Autodesk Inventor part; units mm, degrees
ref_plane "YZ Plane" through (0, 0, 0) normal (1, 0, 0) x (0, 1, 0)
ref_plane "XZ Plane" through (0, 0, 0) normal (0, 1, 0) x (-1, 0, 0)
ref_plane "XY Plane" through (0, 0, 0) normal (0, 0, 1) x (1, 0, 0)
sketch "Boceto1" plane through (0, 0, 0) normal (0, 0, 1) x (1, 0, 0)
  line L0 (0, 0) -> (0, 30.8)
  line L1 (0, 30.8) -> (7, 30.8)
  line L2 (7, 30.8) -> (7, 20.8)
  line L3 (0, 0) -> (45, 0)
  line L4 (45, 0) -> (45, 4.6)
  line L5 (45, 4.6) -> (17, 4.6)
  line L6 (17, 4.6) -> (7, 20.8)
  dimension "d0" = 30.8
  dimension "d1" = 7
  dimension "d2" = 10
  dimension "d3" = 45
  dimension "d4" = 4.6
  dimension "d5" = 28
extrude "Extrusión1" add sketch "Boceto1" along normal blind 1.8
sketch "Boceto2" plane through (0, 0, 1.8) normal (0, 0, 1) x (1, 0, 0)
  line L0 (0, 0) -> (0, 30.8)
  line L1 (45, 0) -> (0, 0)
  line L2 (45, 4.6) -> (45, 0)
  line L3 (17, 4.6) -> (45, 4.6)
  line L4 (7, 30.8) -> (7, 20.8)
  line L5 (17, 4.6) -> (7, 4.6)
  line L6 (0, 6.8) -> (7, 6.8)
  line L7 (7, 6.8) -> (7, 4.6)
  line L8 (0, 30.8) -> (7, 30.8)
  line L9 (7, 30.8) -> (7, 28.8)
  line L10 (7, 28.8) -> (0, 28.8)
  line L11 (0, 28.8) -> (0, 30.8)
  dimension "d8" = 10
  dimension "d14" = 6.8
  dimension "d18" = 2
extrude "Extrusión2" add sketch "Boceto2" along normal blind 2.2
fillet "Empalme1" radius 1 4 edges at (45, 0, 2) (45, 2.3, 0) (45, 4.6, 2) (45, 2.3, 4)
fillet "Empalme2" radius 1 4 edges at (7, 6.8, 2.9) (7, 28.8, 2.9) (12, 12.7, 1.8) (7, 24.8, 1.8)
sketch "Boceto3" plane through (45, 1, 3) normal (1, 0, 0) x (0, 0, -1)
  line L0 (2, 0) -> (0, 0)
  line L1 (2, 2.6) -> (2, 0)
  point P0 (3, -1)
  point P1 (1, 0.5)
  dimension "d20" = 0.5
  dimension "d21" = 1
hole "Hole1" at (45, 1.5, 2) direction (-1, 0, 0) diameter 1 depth 3
equation "\"Radio_pliegue\" = Grosor"
equation "\"Anchura_desahogo_plegado\" = Grosor"
equation "\"Profundidad_desahogo_plegado\" = 0.5 * Grosor"
equation "\"Tamaño_destalonado\" = 4 * Grosor"
equation "\"Remanente_mínimo\" = 2 * Grosor"
equation "\"Radiodetransición\" = Radio_pliegue"
equation "\"Tamaño_de_radio_de_Jacobi\" = Radio_pliegue"
equation "\"TamañoSeparación\" = Grosor"
properties part number "Tirador" material "Por defecto"
Design review of the part built by this model. Coordinates are the model's own, in mm. A direction names the side the tool comes from. Coordinates: 2 decimals unless noted, no trailing zeros. Loops run counter-clockwise (first coordinate to the right, second up) from the corner with the lowest first, then second, coordinate; pieces in that order, holes last. Notation, with made-up numbers: M -26,76.25 L 21,76.25 A17 ccw 21,98.25 Z; hole C 4,52.5 d7. An arc over 180 degrees is marked long. Answer as CSV lines item,"result".
Item 1: Add section C-C on y = 25. State the section outline as (x, z) points, plus the area to 3 significant figures.
Answer list:
outline,"M 0,0 L 7,0 L 7,0.8 A1 ccw 6,1.8 L 0,1.8 Z"
area,"12.4 mm²"
Item 2: Add section A-A on y = 1.5. State the section outline as (x, z) points.
Answer list:
outline,"M 0,0 L 44,0 A1 ccw 45,1 L 45,1.5 L 42,1.5 L 42,2.5 L 45,2.5 L 45,3 A1 ccw 44,4 L 0,4 Z"
Item 3: For probe 1 along Y at (x, z) = (43.2, 2); probe 2 along Z at (x, y) = (43.75, 1.5); probe 3 along Y at (x, z) = (21, 2.7), list the stretches that pass through material, from the lowest coordinate up.
Answer list:
probe 1,"0 to 1, 2 to 4.6"
probe 2,"0 to 1.5, 2.5 to 4"
probe 3,"0 to 4.6"
Item 4: Machinability: for faces 1 (the face through (3, 30, 4)), 2 (the face through (42, 1.5, 2)), 3 (the face through (6.715, 25.093, 1.499)), 4 (the face through (12.07, 12.59, 0.39)), 5 (the face through (3, 6.8, 3)), which of the approach directions +Z, -Z, +X, -X, +Y, -Y give a long, thin tool a straight path to every point of the face, cutting with its end or side? Answer none if there is none.
Answer list:
face 1,"+Z, +X, -X, +Y, -Y"
face 2,"+X"
face 3,"+Z, +X"
face 4,"+Z, -Z, +X, +Y"
face 5,"+Z, +X, -X"
Item 5: The part is to be moulded in two halves that separate along Z. For faces 6 (the face through (44.715, 2.332, 0.301)), 7 (the face through (44.6, 0.2, 2)), 8 (the face through (6, 14, 1.8)), 9 (the face through (43, 2, 2)), say which applies: pulls with the +Z half, pulls with the -Z half, needs draft (parallel to the pull), parting line crosses it, or undercut.
Answer list:
face 6,"pulls with the -Z half"
face 7,"needs draft"
face 8,"pulls with the +Z half"
face 9,"undercut"
Item 6: For P1, Ø8, axis at x = 7.5, y = 11.5, coming from the +Z side; P2, Ø1.3, axis at y = 5, z = 3.5, coming from the +X side; P3, Ø2, axis at x = 8.5, y = 19.5, coming from the +Z side; P4, Ø1.5, axis at y = 22, z = 3, coming from the +X side, all flat-tipped, find the tip position at first contact; note any pin that passes through.
Answer list:
P1,"z = 1.8"
P2,"x = 44.66"
P3,"z = 1.6"
P4,"through"
Item 7: Add section B-B on x = 34. State the section outline as (y, z) points, plus the area to 3 significant figures.
Answer list:
outline,"M 0,0 L 4.6,0 L 4.6,4 L 0,4 Z"
area,"18.4 mm²"
